from build123d import *

# Parameters (mm, degrees)
EXTRUDE_1_DEPTH      = 18
SKETCH_10_W          = 36.784417634
SKETCH_10_H          = 49.551694486
CUT_EXTRUDE_7_DEPTH  = 25
SKETCH_11_W          = 28
SKETCH_11_H          = 46.666666667
EXTRUDE_2_DEPTH      = 35
SKETCH_2_R           = 4
CUT_EXTRUDE_9_DEPTH  = 40
CUT_EXTRUDE_10_DEPTH = 22
CUT_EXTRUDE_11_DEPTH = 28


with BuildPart() as part:
    # 草图1 → 凸台-拉伸1 (new body)
    with BuildSketch(Plane.XY):
        with BuildLine():
            Line((-130.576922015, 14.988928879), (-23.496301019, 19.11044112))
            ThreePointArc((-23.496301019, 19.11044112), (-15.422230188, 21.845348847), (-10.142250191, 28.538042722))
            Line((-10.142250191, 28.538042722), (49.433348919, 177.774006572))
            ThreePointArc((49.433348919, 177.774006572), (68.544423032, 186.290222442), (77.578179631, 167.418276909))
            Line((77.578179631, 167.418276909), (18.950963208, -6.392260437))
            ThreePointArc((18.950963208, -6.392260437), (11.349883724, -16.46754807), (-0.770941638, -19.985135701))
            Line((-0.770941638, -19.985135701), (-130.000001063, -15.000027558))
            ThreePointArc((-130.000001063, -15.000027558), (-144.997253695, -0.28851385), (-130.576922015, 14.988928879))
        make_face()
    extrude(amount=EXTRUDE_1_DEPTH)

    # 草图10 → 切除-拉伸7 (cut, symmetric)
    with BuildSketch(Plane.ZY.offset(130)):
        Rectangle(SKETCH_10_W, SKETCH_10_H)
    extrude(amount=CUT_EXTRUDE_7_DEPTH, both=True, mode=Mode.SUBTRACT)

    # 草图11 → 凸台-拉伸2 (add)
    with BuildSketch(Plane.ZY.offset(105)):
        with Locations((9, 0.004479114)):
            Rectangle(SKETCH_11_W, SKETCH_11_H)
    extrude(amount=EXTRUDE_2_DEPTH)

    # 草图2 → 切除-拉伸9 (cut, symmetric)
    with BuildSketch(Plane.XY):
        with Locations((63.364635235, 172.212580846)):
            Circle(SKETCH_2_R)
        with Locations(Location((-130, 0, 0), (0, 0, 270))):
            Circle(SKETCH_2_R)
    extrude(amount=CUT_EXTRUDE_9_DEPTH, both=True, mode=Mode.SUBTRACT)

    # 草图16 → 切除-拉伸10 (cut)
    with BuildSketch(Plane.ZY.offset(140)):
        Polygon((1, 0), (1, -23.32885422), (17, -23.32885422), (17, 23.337812447), (1, 23.337812447), align=None)
    extrude(amount=-CUT_EXTRUDE_10_DEPTH, mode=Mode.SUBTRACT)

    # 草图17 → 切除-拉伸11 (cut)
    with BuildSketch(Plane(origin=(0, 0, -5), x_dir=(-1, 0, 0), z_dir=(0, 0, -1))):
        with BuildLine():
            Line((118, 23.337812447), (140, 23.337812447))
            Line((140, 23.337812447), (140, -23.32885422))
            Line((140, -23.32885422), (118, -23.337812447))
            Line((118, -23.337812447), (135.587008924, -5.512235317))
            ThreePointArc((135.587008924, -5.512235317), (137.848528965, 0), (135.587008924, 5.512235317))
            Line((135.587008924, 5.512235317), (118, 23.337812447))
        make_face()
    extrude(amount=-CUT_EXTRUDE_11_DEPTH, mode=Mode.SUBTRACT)


solid = part.part
The model under review builds one solid part; all positions refer to its coordinate system, in mm. A direction names the side the tool comes from. Give positions to 0.01 mm unless a question says otherwise; leave off trailing zeros. Loops run counter-clockwise (first coordinate to the right, second up) from the corner with the lowest first, then second, coordinate; pieces in that order, holes last. Notation, with made-up numbers: (14.25, 41.5) -> (19.25, 41.5) arc R27 cw to (19.25, 58.5) -> close; hole circle Ø5 at (73, 79.25). An arc over 180 degrees is marked (long way). Put each result on its own line as item: value. Start each with the question number.
1. We need section A-A on z = -2.5. State the section outline as (x, y) points.
2. For faces 1 (the face through (-52.2, -18, 8.9)), 2 (the face through (-111, 23.338, 9)), 3 (the face through (-125.86, -0.32, 17)), 4 (the face through (-64.82, 17.52, 8.87)), list the 3-axis set-ups (+Z, -Z, +X, -X, +Y, -Y) from which the entire face can be reached by the end or side of a thin tool; tool diameter is ignored.
3. Clearance check with flat-ended pins moving along their axes: P1, Ø12, axis at x = 15, y = 77, coming from the -Z side; P2, Ø3, axis at y = 67.5, z = -1, coming from the -X side; P3, Ø1, axis at y = 75.5, z = 9.5, coming from the -X side. State where each tip first meets the part, or that it passes through.
4. We need section D-D on y = 125. State the section outline as (x, z) points, then the cut area to 3 significant figures.
5. Wall thickness on probe 1 along Z at (x, y) = (-121.5, 18.5); probe 2 along Z at (x, y) = (-31.5, 14.5); probe 3 along X at (y, z) = (-5, 15): over which ranges is each line inside the solid? List them lowest first.
6. We need section C-C on x = -130. State the section outline as (y, z) points.
7. We need section B-B on y = 0. State the section outline as (x, z) points.
8. Mouldability with a two-part tool opening along Z and no side actions: class faces 5 (the face through (-126.034, 0.521, 20.042)), 6 (the face through (1, 53, 18)), 7 (the face through (-125.86, 0.33, 1)) as released by +Z, released by -Z, zero draft, split by the parting line, or undercut.
Determined:
1. outline: (-135.59, -5.51) -> (-118.01, -23.33) -> (-105, -23.33) -> (-105, 23.34) -> (-118, 23.34) -> (-135.59, 5.51) arc R7.85 ccw to start; hole circle Ø8 at (-130, 0)
2. face 1: +Z, -Z, -Y
2. face 2: +Z, -Z, -X, +Y
2. face 3: -X, +Y, -Y
2. face 4: +Z, -Z, +Y
3. P1: z = 0
3. P2: x = 4.97
3. P3: x = 8.41
4. outline: (28.37, 0) -> (63.27, 0) -> (63.27, 18) -> (28.37, 18) -> close
4. area: 628 mm^2
5. probe 1: -5 to 1, 17 to 23
5. probe 2: 0 to 18
5. probe 3: -118 to 19.42
6. outline: (-11.18, -5) -> (-4, -5) -> (-4, 1) -> (-11.18, 1) -> close; (-11.18, 17) -> (-4, 17) -> (-4, 23) -> (-11.18, 23) -> close; (4, -5) -> (11.18, -5) -> (11.18, 1) -> (4, 1) -> close; (4, 17) -> (11.18, 17) -> (11.18, 23) -> (4, 23) -> close
7. outline: (-137.85, -5) -> (-134, -5) -> (-134, 1) -> (-137.85, 1) -> close; (-137.85, 17) -> (-134, 17) -> (-134, 23) -> (-137.85, 23) -> close; (-126, -5) -> (-105, -5) -> (-105, 0) -> (21.11, 0) -> (21.11, 18) -> (-105, 18) -> (-105, 23) -> (-126, 23) -> (-126, 17) -> (-118, 17) -> (-118, 1) -> (-126, 1) -> close
8. face 5: zero draft
8. face 6: released by +Z
8. face 7: undercut
